from build123d import *

# Parameters (mm, degrees)
F0_W     = 100
F0_H     = 100
F1_DEPTH = 100
F3_DEPTH = 100.001
F4_R     = 15
F5_DEPTH = 102.4305039463


with BuildPart() as f1:
    # F0 (on Front) → F1 (new body)
    with BuildSketch(Plane.XZ):
        with Locations((50, 50)):
            Rectangle(F0_W, F0_H)
    extrude(amount=-F1_DEPTH)

    # F2 (on face) → F3 (cut, through all)
    with BuildSketch(Plane.XZ):
        Polygon((40, 110), (40, 100), (100, 50), (110, 50), (110, 110), align=None)
    extrude(amount=-F3_DEPTH, mode=Mode.SUBTRACT)

    # F4 (on face) → F5 (cut, through all)
    with BuildSketch(Plane(origin=(65.5737704918, 0, 78.6885245902), x_dir=(0.7682212796, 0, -0.6401843997), z_dir=(0.6401843997, 0, 0.7682212796))):
        with Locations((6.7104112174, 50)):
            Circle(F4_R)
    extrude(amount=-F5_DEPTH, mode=Mode.SUBTRACT)


solid = f1.part
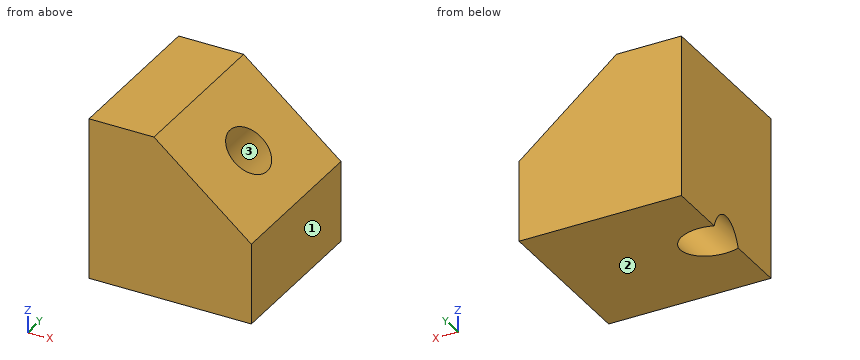
Read the model definition and answer for the solid it produces. Units are mm, in the model's axes. Face numbers are marked on the shaded views. Give positions to 0.01 mm unless a question says otherwise; leave off trailing zeros. Write each loop counter-clockwise with the first axis right and the second up, starting at its lowest first coordinate (ties: lowest second). Pieces come first, ordered by that corner, then holes. Notation, with made-up numbers: (-11, 86) -> (-2, 86) arc R17 ccw to (-2, 102) -> close; hole circle Ø5 at (24.5, 84). An arc over 180 degrees is marked (long way). Answer as a JSON object with one key per item and string values. Group by question number.
1) Find section A-A (y = 47). Write down the section's boundary in (x, z), and give its area (3 significant figures).
2) The mould has two halves that part along X. Classify the marked faces 1, 2 and 3: +X half, -X half, draft (parallel to the pull), parting line (faces both ways), or undercut.
3) Each of these flat-tipped pins is pushed along its axis until it touches: P1, Ø4, axis at x = 54.5, y = 18.5, coming from the +Z side; P2, Ø8, axis at y = 23.5, z = 59.5, coming from the +X side; P3, Ø6, axis at x = 80.5, y = 60, coming from the +Z side; P4, Ø8, axis at y = 36.5, z = 43.5, coming from the -X side. Where does it stop, or does it pass through?
4) Consider L1, parallel to X at y = 49, z = 61; L2, parallel to Y at x = 50, z = 34; L3, parallel to X at y = 47, z = 46. Determine where each line is inside the solid, lowest interval first. Write a range as from..to.
5) Find section B-B (y = 29.5). Write down the section's boundary in (x, z).
Values follow:
{
 "1": {"outline": "(0, 12.48) -> (59.44, 83.8) -> (40, 100) -> (0, 100) -> close; (27.87, 0) -> (100, 0) -> (100, 50) -> (82.02, 64.98) -> close", "area": "5,720 mm2"},
 "2": {"face 1": "+X half", "face 2": "draft", "face 3": "undercut"},
 "3": {"P1": "stops at z = 89.58", "P2": "stops at x = 93.4", "P3": "stops at z = 68.34", "P4": "stops at x = 0"},
 "4": {"L1": "x = 0..40.09, 79.05..86.8", "L2": "y = 0..38.76, 61.24..100", "L3": "x = 0..27.94, 66.2..100"},
 "5": {"outline": "(0, 0) -> (100, 0) -> (100, 50) -> (40, 100) -> (0, 100) -> close"}
}
